Source: CAD feature listing. Evaluate the final solid. Frame: model axes, mm. A direction names the side the tool comes from. Coordinates: 2 decimals unless noted, no trailing zeros. Write each loop counter-clockwise with the first axis right and the second up, starting at its lowest first coordinate (ties: lowest second). Pieces come first, ordered by that corner, then holes. Notation, with made-up numbers: (87.5, -38.75) -> (94.5, -38.75) arc R29 ccw to (94.5, -16.75) -> close; hole circle Ø8 at (-16.75, 82). An arc over 180 degrees is marked (long way). One line per item, written item: value. Start each with the question number.
1. Section query A-A, the plane y = -10.5. Output: boundary loops of the cut face in (x, z).
2. Access query for faces 5 (the cylindrical face through (21.434, -27.621, -11.639)), 6 (the flat face through (-10.17, -6, 11)), 7 (the flat face through (-21, -12.7, 7)). Directions: +Z, -Z, +X, -X, +Y, -Y. A direction counts if a zero-diameter tool reaches every point of the face in a straight line with its end or side. Return the directions, or none.
3. Section query C-C, the plane z = 20.5. Output: boundary loops of the cut face in (x, y), and give its area (3 significant figures).
4. Section query B-B, the plane x = -18. Output: boundary loops of the cut face in (y, z), and give its area (3 significant figures).
5. Section query D-D, the plane y = -5. Output: boundary loops of the cut face in (x, z), and give its area (3 significant figures).
6. Line query: line 1 (X direction, y = -29.5, z = -10); line 2 (Z direction, x = 8, y = -24); line 3 (Z direction, x = -25.5, y = -7). Output: solid intervals per line, ascending.
7. First-contact query: P1, Ø4, axis at x = -23, y = -24.5, coming from the +Z side; P2, Ø11.5, axis at x = -13.5, y = -16, coming from the +Z side; P3, Ø14, axis at y = -5, z = 11.5, coming from the +X side; P4, Ø8.5, axis at x = 18.41, y = -9.52, coming from the -Z side. Flat tips, straight axial feed; report the tip coordinate or a pass-through.
8. Mould query, pull axis Z, two halves, no side actions, for faces 1 (the cylindrical face through (-27.55, -6.439, 21.183)), 2 (the flat face through (-4, -19, -14.858)), 3 (the flat face through (-4, -38.1, -12)), 4 (the flat face through (-4, -24, -8.508)). Classes: released by +Z, released by -Z, zero draft, split by the parting line, or undercut.
from build123d import *

# Parameters (mm, degrees)
F0_W     = 63.5
F0_H     = 44.45
F1_DEPTH = 38.1
F2_W     = 63.5
F2_H     = 38.1
F3_DEPTH = 25.4
F4_R     = 6.35
F5_DEPTH = 12.7
F6_R     = 3.175
F7_DEPTH = 6.35


with BuildPart() as f1:
    # F0 (on Front) → F1 (new body)
    with BuildSketch(Plane.XZ):
        with Locations((-3.8195736706, 7.3665864387)):
            Rectangle(F0_W, F0_H)
    extrude(amount=F1_DEPTH)

    # F2 (on face) → F3 (cut)
    with BuildSketch(Plane.XZ.offset(38.1)):
        with Locations((-3.8195736706, 10.5415864387)):
            Rectangle(F2_W, F2_H)
    extrude(amount=-F3_DEPTH, mode=Mode.SUBTRACT)

    # F4 (on face) → F5 (cut)
    with BuildSketch(Plane.XZ.offset(12.7)):
        with BuildLine():
            Line((-35.5695736706, 29.5915864387), (-35.5695736706, 16.8915864387))
            ThreePointArc((-35.5695736706, 16.8915864387), (-31.8498297917, 25.8718425598), (-22.8695736706, 29.5915864387))
            Line((-22.8695736706, 29.5915864387), (-35.5695736706, 29.5915864387))
        make_face()
        with BuildLine():
            ThreePointArc((-10.1695736706, 4.1915864387), (-6.4498297917, -4.7886696824), (2.5304263294, -8.5084135613))
            Line((2.5304263294, -8.5084135613), (27.9304263294, -8.5084135613))
            Line((27.9304263294, -8.5084135613), (27.9304263294, 29.5915864387))
            Line((27.9304263294, 29.5915864387), (-22.8695736706, 29.5915864387))
            ThreePointArc((-22.8695736706, 29.5915864387), (-13.8893175496, 25.8718425598), (-10.1695736706, 16.8915864387))
            Line((-10.1695736706, 16.8915864387), (-10.1695736706, 4.1915864387))
        make_face()
        with Locations((-22.8695736706, 16.8915864387)):
            Circle(F4_R)
    extrude(amount=-F5_DEPTH, mode=Mode.SUBTRACT)

    # F6 (on face) → F7 (cut)
    with BuildSketch(Plane.XY.offset(-8.5084135613)):
        with Locations((18.4054263294, -9.525)):
            Circle(F6_R)
        with Locations((18.4054263294, -28.575)):
            Circle(F6_R)
        with Locations((-26.0445736706, -28.575)):
            Circle(F6_R)
        with BuildLine():
            Line((-35.5695736706, -38.1), (-26.0445736706, -38.1))
            ThreePointArc((-26.0445736706, -38.1), (-32.1739472484, -34.7043735778), (-35.5695736706, -28.575))
            Line((-35.5695736706, -28.575), (-35.5695736706, -38.1))
        make_face()
        with BuildLine():
            ThreePointArc((27.9304263294, -28.575), (24.5347999072, -34.7043735778), (18.4054263294, -38.1))
            Line((18.4054263294, -38.1), (27.9304263294, -38.1))
            Line((27.9304263294, -38.1), (27.9304263294, -28.575))
        make_face()
    extrude(amount=-F7_DEPTH, mode=Mode.SUBTRACT)


solid = f1.part
Computed values:
1. outline: (-35.57, -14.86) -> (15.38, -14.86) -> (15.38, -8.51) -> (2.53, -8.51) arc R12.7 cw to (-10.17, 4.19) -> (-10.17, 16.89) arc R12.7 ccw to (-35.57, 16.89) -> close; (21.43, -14.86) -> (27.93, -14.86) -> (27.93, -8.51) -> (21.43, -8.51) -> close; hole circle Ø12.7 at (-22.87, 16.89)
2. face 5: +Z, -Z
2. face 6: +Z, +X, +Y, -Y
2. face 7: +Z, +X, -X, -Y
3. outline: (-35.05, -12.7) -> (-28.09, -12.7) -> (-28.09, 0) -> (-35.05, 0) -> close; (-17.64, -12.7) -> (-10.69, -12.7) -> (-10.69, 0) -> (-17.64, 0) -> close
3. area: 177 mm²
4. outline: (-38.1, -14.86) -> (0, -14.86) -> (0, 12.82) -> (-12.7, 12.82) -> (-12.7, -8.51) -> (-38.1, -8.51) -> close; (-12.7, 20.97) -> (0, 20.97) -> (0, 28.62) -> (-12.7, 28.62) -> close
4. area: 610 mm²
5. outline: (-35.57, -14.86) -> (27.93, -14.86) -> (27.93, -8.51) -> (2.53, -8.51) arc R12.7 cw to (-10.17, 4.19) -> (-10.17, 16.89) arc R12.7 ccw to (-35.57, 16.89) -> close; hole circle Ø12.7 at (-22.87, 16.89)
5. area: 1,210 mm²
6. line 1: x = -35.32 to -29.08, -23.01 to 15.37, 21.44 to 27.68
6. line 2: z = -14.86 to -8.51
6. line 3: z = -14.86 to 11.11, 22.67 to 29.32
7. P1: stops at z = -8.51
7. P2: stops at z = 28.71
7. P3: stops at x = -10.17
7. P4: stops at z = -14.86
8. face 1: undercut
8. face 2: released by -Z
8. face 3: zero draft
8. face 4: released by +Z
